from build123d import *

# Parameters (mm, degrees)
EXTRUSION1_DEPTH = 280
ESQUISSE2_R      = 1.5
EXTRUSION2_DEPTH = 282.322324034
ESQUISSE3_R      = 1.5
EXTRUSION3_DEPTH = 10
ESQUISSE4_W      = 18.5
ESQUISSE4_H      = 48.5
ESQUISSE4_H_2    = 21.5
EXTRUSION4_DEPTH = 1.5


with BuildPart() as part:
    # Esquisse1 → Extrusion1 (new body)
    with BuildSketch(Plane.XY):
        Polygon((0, 0), (20, 0), (20, 1.5), (1.5, 1.5), (1.5, 20), (0, 20), align=None)
    extrude(amount=EXTRUSION1_DEPTH)

    # Esquisse2 → Extrusion2 (cut, through all)
    with BuildSketch(Plane(origin=(0, 1.5, 0), x_dir=(1, 0, 0), z_dir=(0, 1, 0))):
        with Locations(Location((12.5, -56, 0), (0, 0, 180))):
            Circle(ESQUISSE2_R)
        with Locations(Location((10, -248.5, 0), (0, 0, 180))):
            Circle(ESQUISSE2_R)
    extrude(amount=-EXTRUSION2_DEPTH, mode=Mode.SUBTRACT)

    # Esquisse3 → Extrusion3 (cut)
    with BuildSketch(Plane.ZY):
        with Locations(Location((268.5, 10, 0), (0, 0, 270))):
            Circle(ESQUISSE3_R)
        with Locations(Location((11.5, 10, 0), (0, 0, 270))):
            Circle(ESQUISSE3_R)
        with Locations(Location((79, 10, 0), (0, 0, 270))):
            Circle(ESQUISSE3_R)
        with Locations(Location((201, 10, 0), (0, 0, 270))):
            Circle(ESQUISSE3_R)
    extrude(amount=-EXTRUSION3_DEPTH, mode=Mode.SUBTRACT)

    # Esquisse4 → Extrusion4 (cut)
    with BuildSketch(Plane.XZ):
        with Locations((10.75, 24.25)):
            Rectangle(ESQUISSE4_W, ESQUISSE4_H)
        with Locations((10.75, 269.25)):
            Rectangle(ESQUISSE4_W, ESQUISSE4_H_2)
    extrude(amount=-EXTRUSION4_DEPTH, mode=Mode.SUBTRACT)


solid = part.part
Could you check a few things on this model? Use its own coordinates, in mm. A direction names the side the tool comes from. Give positions to 0.01 mm unless a question says otherwise; leave off trailing zeros. Order: outer loops, then holes, each group sorted by start corner. A loop starts at its lowest first (then second) coordinate and runs counter-clockwise, first axis right, second up.
1. For faces 1 (the flat face through (11, 1.5, 152)), 2 (the flat face through (10, 0, 138)), which set-ups out of +Z, -Z, +X, -X, +Y, -Y let a thin tool reach every point of the face, with its end or its side?
2. I need wall thicknesses on L1, parallel to Z at x = 1.1, y = 10; L2, parallel to X at y = 0.4, z = 248.5; L3, parallel to Z at x = 10, y = 0.65. Which ranges of each line are inside material? Lowest first, please.
3. Suppose I cut it at A-A (z = 206.5). List the corners of the cut face in (x, y) for me, plus the area to 4 significant figures.
4. Will these pins go through, and if not, where does the flat tip stop? P1, Ø1.6, axis at x = 10, y = 1, coming from the +Z side; P2, Ø4, axis at x = 15, z = 176, coming from the -Y side; P3, Ø5.5, axis at x = 9, z = 162.5, coming from the +Y side; P4, Ø1.8, axis at y = 10, z = 79, coming from the -X side.
5. Suppose I cut it at B-B (x = 5). List the corners of the cut face in (y, z) for me, plus the area to 3 significant figures.
6. Suppose I cut it at C-C (y = 4). List the corners of the cut face in (x, z) for me.
Solved:
1. face 1: +Z, -Z, +X, +Y
1. face 2: +Z, -Z, +X, -X, -Y
2. L1: z = 0 to 10, 13 to 77.5, 80.5 to 199.5, 202.5 to 267, 270 to 280
2. L2: x = 0 to 8.5, 11.5 to 20
2. L3: z = 48.5 to 247, 250 to 258.5
3. outline: (0, 0) - (20, 0) - (20, 1.5) - (1.5, 1.5) - (1.5, 20) - (0, 20) - close
3. area: 57.75 mm2
4. P1: stops at z = 258.5
4. P2: stops at y = 0
4. P3: stops at y = 1.5
4. P4: passes through
5. outline: (0, 48.5) - (1.5, 48.5) - (1.5, 258.5) - (0, 258.5) - close
5. area: 315 mm2
6. outline: (0, 0) - (1.5, 0) - (1.5, 280) - (0, 280) - close
